from build123d import *
from build123d.topology import SkipClean

# Parameters (mm, degrees)
SKETCH1_R              = 330.20000000000005
BOSS_EXTRUDE1_DEPTH    = 889
SKETCH2_R              = 304.8
CUT_EXTRUDE1_DEPTH     = 876.3
SKETCH5_R              = 381
BOSS_EXTRUDE2_DEPTH    = 50.8
CUT_EXTRUDE2_START     = -1e-07
CUT_EXTRUDE2_OUTLINE_R = 304.8
CUT_EXTRUDE2_DEPTH     = 889.0000002


with BuildPart() as part:
    # Sketch1 → Boss-Extrude1 (new body)
    with BuildSketch(Plane(origin=(0, 0, 0), x_dir=(1, 0, 0), z_dir=(0, 1, 0))):
        with Locations(Location((0, 0, 0), (0, 0, 270))):
            Circle(SKETCH1_R)
    extrude(amount=BOSS_EXTRUDE1_DEPTH)

    # Sketch2 → Cut-Extrude1 (cut)
    with BuildSketch(Plane(origin=(0, 889, 0), x_dir=(1, 0, 0), z_dir=(0, 1, 0))):
        with Locations(Location((0, 0, 0), (0, 0, 270))):
            Circle(SKETCH2_R)
    extrude(amount=-CUT_EXTRUDE1_DEPTH, mode=Mode.SUBTRACT)

    # Sketch5 → Boss-Extrude2 (add)
    with BuildSketch(Plane.XZ):
        with Locations(Location((0, 0, 0), (0, 0, 270))):
            Circle(SKETCH5_R)
    extrude(amount=-BOSS_EXTRUDE2_DEPTH)

    # Sketch8 → Revolve1 (revolve)
    with BuildSketch(Plane.XZ):
        with BuildLine():
            Line((330.2, 0), (-330.2, 0))
            ThreePointArc((-330.2, 0), (2.022e-14, 330.2), (330.2, 0))
        make_face()
    revolve(axis=Axis((330.2, 0, 0), (-1, 0, 0)))

    # Sketch11 → Cut-Revolve1 (revolve, cut)
    with BuildSketch(Plane(origin=(0, 0, 0), x_dir=(1, 0, 0), z_dir=(0, 1, 0))):
        with BuildLine():
            Line((304.80000000000007, 0), (-304.80000000000007, 0))
            ThreePointArc((-304.80000000000007, 0), (1.866e-14, 304.80000000000007), (304.80000000000007, 0))
        make_face()
    revolve(axis=Axis((304.80000000000007, 0, 0), (-1, 0, 0)), mode=Mode.SUBTRACT)

    # Cut-Extrude2: read off the stored shape, not the designer's step
    # Cut-Extrude2 outline → Cut-Extrude2 (cut)
    with SkipClean():  # the faces are left unmerged after this step: merging them gives an invalid solid
        with BuildSketch(Plane(origin=(0, 0, 0), x_dir=(1, 0, 0), z_dir=(0, 1, 0)).offset(CUT_EXTRUDE2_START)):
            Circle(CUT_EXTRUDE2_OUTLINE_R)
        extrude(amount=CUT_EXTRUDE2_DEPTH, mode=Mode.SUBTRACT)

    # Sketch14 → Loft3 section 0
    with SkipClean():  # the faces are left unmerged after this step: merging them gives an invalid solid
        with BuildSketch(Plane(origin=(0, 0, 0), x_dir=(1, 0, 0), z_dir=(0, 1, 0))):
            with BuildLine():
                Line((-22.260323000361307, -330.2), (28.53967699963869, -330.2))
                Line((28.53967699963869, -330.2), (28.53967699963869, -279.4))
                Line((28.53967699963869, -279.4), (-22.260323000361307, -279.4))
                Line((-22.260323000361307, -279.4), (-22.260323000361307, -330.2))
            make_face()
        # Sketch17 → Loft3 section 1
        with BuildSketch(Plane(origin=(0, -1143, 0), x_dir=(1, 0, 0), z_dir=(0, 1, 0))):
            with BuildLine():
                Line((-28.71955564169997, -533.4000000000001), (22.08044435830003, -533.4000000000001))
                Line((22.08044435830003, -533.4000000000001), (22.080444358300024, -482.6))
                Line((22.080444358300024, -482.6), (-28.71955564169998, -482.6))
                Line((-28.71955564169998, -482.6), (-28.71955564169997, -533.4000000000001))
            make_face()
        loft()

    # Sketch14<7> → Loft4 section 0
    with SkipClean():  # the faces are left unmerged after this step: merging them gives an invalid solid
        with BuildSketch(Plane(origin=(0, 0, 0), x_dir=(1, 0, 0), z_dir=(0, 1, 0))):
            with BuildLine():
                Line((279.4, -19.993284341920333), (330.2, -19.993284341920333))
                Line((330.2, -19.993284341920333), (330.2, 30.806715658079664))
                Line((330.2, 30.806715658079664), (279.4, 30.806715658079664))
                Line((279.4, 30.806715658079664), (279.4, -19.993284341920333))
            make_face()
        # Sketch17<4> → Loft4 section 1
        with BuildSketch(Plane(origin=(0, -1143, 0), x_dir=(1, 0, 0), z_dir=(0, 1, 0))):
            with BuildLine():
                Line((482.5999999999999, -25.4), (533.3999999999999, -25.4))
                Line((533.3999999999999, -25.4), (533.3999999999999, 25.4))
                Line((533.3999999999999, 25.4), (482.5999999999999, 25.4))
                Line((482.5999999999999, 25.4), (482.5999999999999, -25.4))
            make_face()
        loft()

    # Sketch14<8> → Loft5 section 0
    with SkipClean():  # the faces are left unmerged after this step: merging them gives an invalid solid
        with BuildSketch(Plane(origin=(0, 0, 0), x_dir=(1, 0, 0), z_dir=(0, 1, 0))):
            with BuildLine():
                Line((-28.539676999638676, 279.4), (22.260323000361325, 279.4))
                Line((22.260323000361325, 279.4), (22.26032300036131, 330.2))
                Line((22.26032300036131, 330.2), (-28.539676999638687, 330.2))
                Line((-28.539676999638687, 330.2), (-28.539676999638676, 279.4))
            make_face()
        # Sketch17<5> → Loft5 section 1
        with BuildSketch(Plane(origin=(0, -1143, 0), x_dir=(1, 0, 0), z_dir=(0, 1, 0))):
            with BuildLine():
                Line((-28.71955564169995, 482.59999999999997), (22.080444358300046, 482.59999999999997))
                Line((22.080444358300046, 482.59999999999997), (22.08044435830004, 533.4))
                Line((22.08044435830004, 533.4), (-28.71955564169996, 533.4))
                Line((-28.71955564169996, 533.4), (-28.71955564169995, 482.59999999999997))
            make_face()
        loft()

    # Sketch17<6> → Loft6 section 0
    with SkipClean():  # the faces are left unmerged after this step: merging them gives an invalid solid
        with BuildSketch(Plane(origin=(0, -1143, 0), x_dir=(1, 0, 0), z_dir=(0, 1, 0))):
            with BuildLine():
                Line((-482.59999999999997, -35.064827171702525), (-533.4, -35.06482717170253))
                Line((-533.4, -35.06482717170253), (-533.4, 15.735172828297465))
                Line((-533.4, 15.735172828297465), (-482.59999999999997, 15.73517282829747))
                Line((-482.59999999999997, 15.73517282829747), (-482.59999999999997, -35.064827171702525))
            make_face()
        # Sketch14<9> → Loft6 section 1
        with BuildSketch(Plane(origin=(0, 0, 0), x_dir=(1, 0, 0), z_dir=(0, 1, 0))):
            with BuildLine():
                Line((-330.20000000000005, -30.75867207748477), (-279.40000000000003, -30.75867207748477))
                Line((-279.40000000000003, -30.75867207748477), (-279.40000000000003, 20.041327922515226))
                Line((-279.40000000000003, 20.041327922515226), (-330.20000000000005, 20.041327922515226))
                Line((-330.20000000000005, 20.041327922515226), (-330.20000000000005, -30.75867207748477))
            make_face()
        loft()


solid = part.part
Verification items for the finished model (mm, model axes). A direction names the side the tool comes from. Coordinates: 2 decimals unless noted, no trailing zeros. Loops run counter-clockwise (first coordinate to the right, second up) from the corner with the lowest first, then second, coordinate; pieces in that order, holes last. Notation, with made-up numbers: (-4, 78) -> (17, 78) arc R4 ccw to (17, 84) -> close; hole circle Ø4 at (-38.75, -38.5). An arc over 180 degrees is marked (long way). Write each question's results on one line, items separated by ' | '.
Item 1: Material ranges on L1, parallel to X at y = 577, z = 0; L2, parallel to Z at x = -22, y = 766.5 (3 decimals), recorded low to high.
Found:
L1: x = -330.2 to -304.8, 304.8 to 330.2 | L2: z = -329.466 to -304.005, 304.005 to 329.466
Item 2: Section check D-D, the plane y = -619. Count the separate pieces of the cut face and the enclosed holes in it, plus the area to 3 significant figures.
Found:
separate pieces: 4 | enclosed holes: 0 | area: 10,300 mm2
Item 3: Gauge pin test, flat ends, axial feed: pin 1 (7.5 mm diameter, centred on x = -288.5, z = 15.5, fed in from +Y); pin 2 (8 mm diameter, centred on x = 85, y = 176.5, fed in from +Z); pin 3 (8 mm diameter, centred on x = 95.5, z = 107, fed in from +Y). Record the tip position at first contact, or that the pin passes through.
Found:
pin 1: stops at y = 0 | pin 2: stops at z = 320.11 | pin 3: stops at y = -266.78
Item 4: Section check B-B, the plane x = 88. Enter the section's corners in (y, z), plus the area to 3 significant figures.
Found:
outline: (0, -370.7) -> (50.8, -370.7) -> (50.8, -318.26) -> (889, -318.26) -> (889, -291.82) -> (0, -291.82) arc R291.82 cw to (0, 291.82) -> (889, 291.82) -> (889, 318.26) -> (50.8, 318.26) -> (50.8, 370.7) -> (0, 370.7) -> (0, 318.26) arc R318.26 ccw to (0, -318.26) -> close | area: 77,700 mm2
Item 5: Section check A-A, the plane y = 218. Enter the section's corners in (x, z).
Found:
outline: circle Ø660.4 at (0, 0); hole circle Ø609.6 at (0, 0)
Item 6: Tool access check on faces 1 (the face through (-508, -1143, 10)), 2 (the face through (327.39, 464.03, -42.99)). Record the directions out of +Z, -Z, +X, -X, +Y, -Y that give a thin tool (end or side, any length) a straight path to the whole face; none if there is none.
Found:
face 1: +Z, -Z, +X, -X, -Y | face 2: +Y
Item 7: Section check C-C, the plane z = 237.5. Enter the section's corners in (x, y).
Found:
outline: (-297.92, 0) -> (-229.4, 0) arc R229.4 ccw to (229.4, 0) -> (297.92, 0) -> (297.92, 50.8) -> (229.4, 50.8) -> (229.4, 889) -> (191.04, 889) -> (191.04, 0) arc R191.04 cw to (-191.04, 0) -> (-191.04, 889) -> (-229.4, 889) -> (-229.4, 50.8) -> (-297.92, 50.8) -> close
